Check sheet for the modelled part. Datum: model origin and axes. Units: mm. A direction names the side the tool comes from. Round coordinates to 2 decimals unless told otherwise and drop trailing zeros. Write each loop counter-clockwise with the first axis right and the second up, starting at its lowest first coordinate (ties: lowest second). Pieces come first, ordered by that corner, then holes. Notation, with made-up numbers: (27.25, 26) - (64.25, 26) arc R5 cw to (64.25, 35) - close; hole circle Ø5 at (-34.5, 15). An arc over 180 degrees is marked (long way). Answer as a JSON object with one key per item and string values. Group by question number.
Item 1: Set-up check for faces 1 (the cylindrical face through (-7.493, 0.493, 0.33)), 2 (the flat face through (-2, 0, -7.4)): record each of +Z, -Z, +X, -X, +Y, -Y from which the full face is reachable in a straight line by a thin tool's end or side.
Item 2: Sectioned sample at B-B on y = 33. Record the boundary of the cut face in (x, z).
Item 3: Thickness scan on line 1 (Z direction, x = 0, y = 32); line 2 (Z direction, x = 0, y = 0.5); line 3 (Y direction, x = 2.5, z = -3.25). Record the ranges inside material, lowest first.
Item 4: Sectioned sample at C-C on x = 0. Record the boundary of the cut face in (y, z).
Item 5: Sectioned sample at D-D on y = 59.5. Record the boundary of the cut face in (x, z), plus the area to 3 significant figures.
Item 6: Gauge pin test, flat ends, axial feed: P1, Ø0.9, axis at x = 0.5, z = 0.5, coming from the -Y side; P2, Ø3.5, axis at x = 0, z = 0, coming from the -Y side; P3, Ø1.5, axis at x = -2.5, z = 3, coming from the -Y side. Record the tip position at first contact, or that the pin passes through.
Item 7: Sectioned sample at A-A on z = 0. Record the boundary of the cut face in (x, y), plus the area to 3 significant figures.
Item 8: Release check for a two-part mould opening along Z. For faces 3 (the flat face through (0, 70, 0)), 4 (the flat face through (-2, 1, 2)), 5 (the cylindrical face through (-1.172, 34.51, -8.923)) record: pulls with the +Z half, pulls with the -Z half, needs draft (parallel to the pull), parting line crosses it, or undercut.
```python
from build123d import *

# Parameters (mm, degrees)
SKETCH2_R           = 9
BOSS_EXTRUDE1_DEPTH = 70
SKETCH3_R           = 7.5
CUT_EXTRUDE1_DEPTH  = 1
SKETCH4_R           = 1.5
CUT_EXTRUDE2_DEPTH  = 50
CHAMFER1_SIZE       = 1
CHAMFER1_SIZE2      = 1.732050808


with BuildPart() as part:
    # Sketch2 → Boss-Extrude1 (new body)
    with BuildSketch(Plane(origin=(0, 0, 0), x_dir=(1, 0, 0), z_dir=(0, 1, 0))):
        Circle(SKETCH2_R)
    extrude(amount=BOSS_EXTRUDE1_DEPTH)

    # Sketch3 → Cut-Extrude1 (cut)
    with BuildSketch(Plane.XZ):
        Circle(SKETCH3_R)
    extrude(amount=-CUT_EXTRUDE1_DEPTH, mode=Mode.SUBTRACT)

    # Sketch4 → Cut-Extrude2 (cut)
    with BuildSketch(Plane.XZ.offset(-1)):
        Circle(SKETCH4_R)
    extrude(amount=-CUT_EXTRUDE2_DEPTH, mode=Mode.SUBTRACT)

    # Chamfer1
    chamfer1_edges = [part.edges().sort_by_distance(p)[0] for p in [
        (-1.5, 1, 0),
    ]]
    chamfer1_side = [part.faces().sort_by_distance(p)[0] for p in [
        (-7.287867966, 1, 0),
    ]]
    chamfer(chamfer1_edges, length=CHAMFER1_SIZE, length2=CHAMFER1_SIZE2, reference=chamfer1_side[0])


solid = part.part
```
Completed:
{
 "1": {"face 1": "-Y", "face 2": "+Z, -Z, +X, -X, -Y"},
 "2": {"outline": "circle Ø18 at (0, 0); hole circle Ø3 at (0, 0)"},
 "3": {"line 1": "-9 to -1.5, 1.5 to 9", "line 2": "-9 to -7.5, 7.5 to 9", "line 3": "1 to 70"},
 "4": {"outline": "(0, -9) - (70, -9) - (70, 9) - (0, 9) - (0, 7.5) - (1, 7.5) - (1, 2.5) - (2.73, 1.5) - (51, 1.5) - (51, -1.5) - (2.73, -1.5) - (1, -2.5) - (1, -7.5) - (0, -7.5) - close"},
 "5": {"outline": "circle Ø18 at (0, 0)", "area": "254 mm²"},
 "6": {"P1": "y = 51", "P2": "y = 2.3", "P3": "y = 1"},
 "7": {"outline": "(-9, 0) - (-7.5, 0) - (-7.5, 1) - (-2.5, 1) - (-1.5, 2.73) - (-1.5, 51) - (1.5, 51) - (1.5, 2.73) - (2.5, 1) - (7.5, 1) - (7.5, 0) - (9, 0) - (9, 70) - (-9, 70) - close", "area": "1,090 mm²"},
 "8": {"face 3": "needs draft", "face 4": "undercut", "face 5": "parting line crosses it"}
}
